Build history of the part. All positions in model axes, mm. A direction names the side the tool comes from. Give positions to 0.01 mm unless a question says otherwise; leave off trailing zeros. Write each loop counter-clockwise with the first axis right and the second up, starting at its lowest first coordinate (ties: lowest second). Pieces come first, ordered by that corner, then holes. Notation, with made-up numbers: (75.5, -23) -> (119.5, -23) arc R33 ccw to (119.5, 9) -> close; hole circle Ø6 at (25, 11). An arc over 180 degrees is marked (long way). One line per question, with ' | ' between items. Start each with the question number.
(1) Tool access for faces 1 (the flat face through (-22.817, -37, 28)), 2 (the flat face through (-1, 0, -9)): list every direction of +Z, -Z, +X, -X, +Y, -Y with a clear straight run to the whole face (end or side of a thin tool).
(2) Drill centre lines: probe 1 along X at (y, z) = (-34, 30); probe 2 along Z at (x, y) = (9.5, -63). Where is each one in solid material? Low to high. Write a range as from..to.
(3) Band-saw the part on C-C, the plane x = 6. Give the cut face in (y, z).
(4) Band-saw the part on B-B, the plane z = 10. Give the cut face in (x, y).
(5) Pull direction X, two halves, no side cores. Call faces 3 (the flat face through (33, -37, 56.017)), 4 (the flat face through (-42.87, -37, -11)), 5 (the flat face through (22.817, -37, 28)): released by +X, released by -X, zero draft, split by the parting line, or undercut.
(6) Pin check, flat tip, straight feed: P1, Ø2, axis at x = -6, y = -29, coming from the +Z side. Stop position of the tip, or through.
(7) Band-saw the part on A-A, the plane y = -9.5. Give the cut face in (x, z), and give its area (3 significant figures).
from build123d import *

# Parameters (mm, degrees)
F0_W     = 20.052685
F0_H     = 56.016997
F1_DEPTH = 75.946


with BuildPart() as f1:
    # F0 (on Front) → F1 (new body)
    with BuildSketch(Plane.XZ):
        Polygon((22.817267, 0), (0, 0), (0, -22.313809), (42.869952, -22.313809), (42.869952, 0), align=None)
        Polygon((0, -22.313809), (0, 0), (-22.817267, 0), (-42.869952, 0), (-42.869952, -22.313809), align=None)
        with Locations((32.843609, 28.008498)):
            Rectangle(F0_W, F0_H)
        with Locations((-32.843609, 28.008498)):
            Rectangle(F0_W, F0_H)
    extrude(amount=F1_DEPTH)


solid = f1.part
Results:
1) face 1: +Z, +Y, -Y | face 2: +Z, -Z, +X, -X, +Y
2) probe 1: x = -42.87..-22.82, 22.82..42.87 | probe 2: z = -22.31..0
3) outline: (-75.95, -22.31) -> (0, -22.31) -> (0, 0) -> (-75.95, 0) -> close
4) outline: (-42.87, -75.95) -> (-22.82, -75.95) -> (-22.82, 0) -> (-42.87, 0) -> close; (22.82, -75.95) -> (42.87, -75.95) -> (42.87, 0) -> (22.82, 0) -> close
5) face 3: zero draft | face 4: released by -X | face 5: undercut
6) P1: stops at z = 0
7) outline: (-42.87, -22.31) -> (42.87, -22.31) -> (42.87, 56.02) -> (22.82, 56.02) -> (22.82, 0) -> (-22.82, 0) -> (-22.82, 56.02) -> (-42.87, 56.02) -> close | area: 4,160 mm²
